```python
from build123d import *

# Parameters (mm, degrees)
BOSS_EXTRUDE1_DEPTH = 6.5
SKETCH4_R           = 1.55
CUT_EXTRUDE1_DEPTH  = 10
SKETCH5_R           = 1.55
CUT_EXTRUDE2_DEPTH  = 10


with BuildPart() as part:
    # Sketch3 → Boss-Extrude1 (new body, symmetric)
    with BuildSketch(Plane.XY):
        Polygon((3.175, -3.175), (-4.7625, -3.175), (-4.7625, -4.7625), (4.7625, -4.7625), (4.7625, 4.7625), (3.175, 4.7625), align=None)
    extrude(amount=BOSS_EXTRUDE1_DEPTH, both=True)

    # Sketch4 → Cut-Extrude1 (cut)
    with BuildSketch(Plane(origin=(4.7625, 0, 0), x_dir=(0, 0, -1), z_dir=(1, 0, 0))):
        with Locations((-3, 1.2375)):
            Circle(SKETCH4_R)
    extrude(amount=-CUT_EXTRUDE1_DEPTH, mode=Mode.SUBTRACT)

    # Sketch5 → Cut-Extrude2 (cut)
    with BuildSketch(Plane.XZ.offset(4.7625)):
        with Locations((-1.2375, -3)):
            Circle(SKETCH5_R)
    extrude(amount=-CUT_EXTRUDE2_DEPTH, mode=Mode.SUBTRACT)


solid = part.part
```
Can you work these out from the model? Positions are in its coordinate system, mm. A direction names the side the tool comes from. Give positions to 0.01 mm unless a question says otherwise; leave off trailing zeros. Write each loop counter-clockwise with the first axis right and the second up, starting at its lowest first coordinate (ties: lowest second). Pieces come first, ordered by that corner, then holes. Notation, with made-up numbers: (50, -12) -> (88, -12) arc R13 ccw to (88, 5) -> close; hole circle Ø5 at (-10.5, -10). An arc over 180 degrees is marked (long way). One line per item, written item: value.
Q1. Imagine slicing it at C-C on y = 2.25. Please give me the cut outline in (x, z) (1 decimal).
Results found:
outline: (3.2, -6.5) -> (4.8, -6.5) -> (4.8, 1.8) -> (3.2, 1.8) -> close; (3.2, 4.2) -> (4.8, 4.2) -> (4.8, 6.5) -> (3.2, 6.5) -> close
Q2. Please list where these lines run through material, in increasing order: line 1 (Y direction, x = 4.2, z = 3); line 2 (X direction, y = 2.5, z = 5) (1 decimal); line 3 (Y direction, x = -0.5, z = 5.25) (1 decimal). Write a range as [from, to].
Results found:
line 1: y = [-4.76, -0.31], [2.79, 4.76]
line 2: x = [3.2, 4.8]
line 3: y = [-4.8, -3.2]
Q3. Imagine slicing it at A-A on z = 3. Please give me the cut outline in (x, y) (1 decimal).
Results found:
outline: (-4.8, -4.8) -> (4.8, -4.8) -> (4.8, -0.3) -> (3.2, -0.3) -> (3.2, -3.2) -> (-4.8, -3.2) -> close; (3.2, 2.8) -> (4.8, 2.8) -> (4.8, 4.8) -> (3.2, 4.8) -> close
Q4. We'd pull the mould along Z, two halves only. Please class faces 3 (the face through (4, -2, 6.5)), 4 (the face through (0, -4.762, 0)), 5 (the face through (-0.522, -3.98, -4.375)): +Z half, -Z half, draft (parallel to the pull), parting line (faces both ways), or undercut.
Results found:
face 3: +Z half
face 4: draft
face 5: undercut
Q5. Which directions (+Z, -Z, +X, -X, +Y, -Y) give clear straight access to the entire face, cutting with the end or side of a thin tool? Please do faces 1 (the face through (-1, -3.175, 0)), 2 (the face through (4, 4.762, 0)).
Results found:
face 1: +Z, -Z, -X, +Y
face 2: +Z, -Z, +X, -X, +Y
Q6. For P1, Ø5, axis at x = -1.5, z = 2.5, coming from the +Y side (3 decimals); P2, Ø5, axis at y = 3, z = -5, coming from the -X side (3 decimals); P3, Ø1.9, axis at x = -1.24, z = -3, coming from the +Y side, each with a flat end and sliding along its axis, tell me the tip position at first contact or that it passes through.
Results found:
P1: stops at y = -3.175
P2: stops at x = 3.175
P3: passes through
Q7. Imagine slicing it at D-D on z = -4.75. Please give me the cut outline in (x, y) (1 decimal).
Results found:
outline: (-4.8, -4.8) -> (4.8, -4.8) -> (4.8, 4.8) -> (3.2, 4.8) -> (3.2, -3.2) -> (-4.8, -3.2) -> close
Q8. Imagine slicing it at B-B on y = -4. Please give me the cut outline in (x, z).
Results found:
outline: (-4.76, -6.5) -> (4.76, -6.5) -> (4.76, 6.5) -> (-4.76, 6.5) -> close; hole circle Ø3.1 at (-1.24, -3)
